Geometry check sheet. Reference: the model listing, model coordinates, mm. Face numbers are marked on the shaded views. A direction names the side the tool comes from. Round coordinates to 2 decimals unless told otherwise and drop trailing zeros. Loops run counter-clockwise (first coordinate to the right, second up) from the corner with the lowest first, then second, coordinate; pieces in that order, holes last.
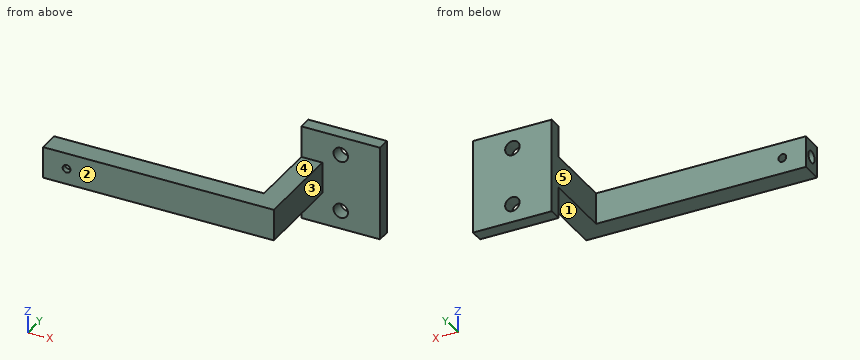
```python
from build123d import *

# Parameters (mm, degrees)
BOSS_EXTRUDE1_DEPTH = 12
SKETCH2_R           = 1.5
CUT_EXTRUDE1_DEPTH  = 12
SKETCH3_R           = 2.25
CUT_EXTRUDE2_DEPTH  = 9
SKETCH4_W           = 36
SKETCH4_H           = 5
BOSS_EXTRUDE2_DEPTH = 30
SKETCH5_R           = 2.75
CUT_EXTRUDE3_DEPTH  = 30


with BuildPart() as part:
    # Sketch1 → Boss-Extrude1 (new body)
    with BuildSketch(Plane.XY):
        Polygon((0, 0), (0, 40), (-8, 40), (-8, 8), (-88, 8), (-88, 0), align=None)
    extrude(amount=BOSS_EXTRUDE1_DEPTH)

    # Sketch2 → Cut-Extrude1 (cut)
    with BuildSketch(Plane(origin=(0, 8, 0), x_dir=(1, 0, 0), z_dir=(0, 1, 0))):
        with Locations(Location((-79, -6, 0), (0, 0, 180))):
            Circle(SKETCH2_R)
    extrude(amount=-CUT_EXTRUDE1_DEPTH, mode=Mode.SUBTRACT)

    # Sketch3 → Cut-Extrude2 (cut)
    with BuildSketch(Plane.ZY.offset(88)):
        with Locations((6, 4)):
            Circle(SKETCH3_R)
    extrude(amount=-CUT_EXTRUDE2_DEPTH, mode=Mode.SUBTRACT)

    # Sketch4 → Boss-Extrude2 (add)
    with BuildSketch(Plane(origin=(-8, 0, 0), x_dir=(0, 0, -1), z_dir=(1, 0, 0))):
        with Locations((-6, 37.5)):
            Rectangle(SKETCH4_W, SKETCH4_H)
    extrude(amount=BOSS_EXTRUDE2_DEPTH)

    # Sketch5 → Cut-Extrude3 (cut)
    with BuildSketch(Plane(origin=(0, 40, 0), x_dir=(1, 0, 0), z_dir=(0, 1, 0))):
        with Locations(Location((7, -17, 0), (0, 0, 180))):
            Circle(SKETCH5_R)
        with Locations(Location((7, 5, 0), (0, 0, 180))):
            Circle(SKETCH5_R)
    extrude(amount=-CUT_EXTRUDE3_DEPTH, mode=Mode.SUBTRACT)


solid = part.part
```
1) Access from +Z, -Z, +X, -X, +Y, -Y to the whole of each face (thin tool, end or side, straight path). Record for the marked faces 1, 2, 3, 4 and 5.
Report:
face 1: -Z, +X, -X, -Y
face 2: +Z, -Z, +X, -X, -Y
face 3: +Z, -Z, +X, -Y
face 4: +Z, +X, -X, -Y
face 5: +Z, -Z, -X, +Y
2) Gauge pin test, flat ends, axial feed: pin 1 (2 mm diameter, centred on x = -6, z = 16.5, fed in from -Y); pin 2 (8 mm diameter, centred on x = -45.5, z = 17, fed in from -Y); pin 3 (0.6 mm diameter, centred on y = 4.5, z = 7.5, fed in from -X); pin 4 (6 mm diameter, centred on x = -35, z = 4, fed in from +Y). Record the tip position at first contact, or that the pin passes through.
Report:
pin 1: stops at y = 35
pin 2: passes through
pin 3: stops at x = -79
pin 4: stops at y = 8
3) Sectioned sample at D-D, the plane y = 4. Record the cut outline in (x, z), then the cut area to 3 significant figures.
Report:
outline: (-88, 0) - (0, 0) - (0, 12) - (-88, 12) - (-88, 8.25) - (-79, 8.25) - (-79, 7.5) arc R1.5 cw to (-79, 4.5) - (-79, 3.75) - (-88, 3.75) - close
area: 1,010 mm2
4) Sectioned sample at C-C, the plane x = 7. Record the cut outline in (y, z), then the cut area to 3 significant figures.
Report:
outline: (35, -12) - (40, -12) - (40, -7.75) - (35, -7.75) - close; (35, -2.25) - (40, -2.25) - (40, 14.25) - (35, 14.25) - close; (35, 19.75) - (40, 19.75) - (40, 24) - (35, 24) - close
area: 125 mm2
5) Scan lines: line 1 along Z through (x, y) = (7, 37); line 2 along Y through (x, z) = (-82, 6); line 3 along Z through (x, y) = (-86, 4). Record each from-to range of solid material in increasing order.
Report:
line 1: z = -12 to -7.75, -2.25 to 14.25, 19.75 to 24
line 2: y = 0 to 1.75, 6.25 to 8
line 3: z = 0 to 3.75, 8.25 to 12
6) Sectioned sample at B-B, the plane z = 6. Record the cut outline in (x, y).
Report:
outline: (-88, 0) - (-80.5, 0) - (-80.5, 1.75) - (-88, 1.75) - close; (-88, 6.25) - (-80.5, 6.25) - (-80.5, 8) - (-88, 8) - close; (-77.5, 0) - (0, 0) - (0, 35) - (22, 35) - (22, 40) - (-8, 40) - (-8, 8) - (-77.5, 8) - close
7) Sectioned sample at A-A, the plane z = 17. Record the cut outline in (x, y).
Report:
outline: (-8, 35) - (4.25, 35) - (4.25, 40) - (-8, 40) - close; (9.75, 35) - (22, 35) - (22, 40) - (9.75, 40) - close
